Input: part model. Units: mm. Frame: model coordinates. A direction names the side the tool comes from. Round coordinates to 2 decimals unless told otherwise and drop trailing zeros. Write each loop counter-clockwise with the first axis right and the second up, starting at its lowest first coordinate (ties: lowest second). Pieces come first, ordered by that corner, then holes. Notation, with made-up numbers: (5.5, 72) -> (32.5, 72) arc R34 cw to (32.5, 102) -> close; hole circle Ø8 at (-26.75, 72.25). An arc over 180 degrees is marked (long way). Use CSV: the item, a comma, the result in double quotes.
```python
from build123d import *

# Parameters (mm, degrees)
CROQUIS1_W              = 90
CROQUIS1_H              = 53
SALIENTE_EXTRUIR1_DEPTH = 3
CROQUIS2_R              = 1.75
CORTAR_EXTRUIR1_DEPTH   = 53.309177015
CROQUIS3_R              = 3.5
CROQUIS3_R_2            = 1.75
SALIENTE_EXTRUIR2_DEPTH = 3
REDONDEO1_R             = 3
CORTAR_EXTRUIR2_DEPTH   = 53.566624392


with BuildPart() as part:
    # Croquis1 → Saliente-Extruir1 (new body)
    with BuildSketch(Plane(origin=(0, 0, 0), x_dir=(1, 0, 0), z_dir=(0, 1, 0))):
        Rectangle(CROQUIS1_W, CROQUIS1_H)
    extrude(amount=SALIENTE_EXTRUIR1_DEPTH)

    # Croquis2 → Cortar-Extruir1 (cut, through all)
    with BuildSketch(Plane.XZ):
        with Locations(Location((41, -22.5, 0), (0, 0, 270))):
            Circle(CROQUIS2_R)
        with Locations(Location((41, 22.5, 0), (0, 0, 270))):
            Circle(CROQUIS2_R)
        with Locations(Location((-41, 22.5, 0), (0, 0, 270))):
            Circle(CROQUIS2_R)
        with Locations(Location((-41, -22.5, 0), (0, 0, 270))):
            Circle(CROQUIS2_R)
    extrude(amount=-CORTAR_EXTRUIR1_DEPTH, mode=Mode.SUBTRACT)

    # Croquis3 → Saliente-Extruir2 (add)
    # profile 1 of 2: a face of its own
    with BuildSketch(Plane(origin=(0, 3, 0), x_dir=(1, 0, 0), z_dir=(0, 1, 0))):
        with Locations(Location((41, 22.5, 0), (0, 0, 270))):
            Circle(CROQUIS3_R)
        with Locations(Location((41, 22.5, 0), (0, 0, 90))):
            Circle(CROQUIS3_R_2, mode=Mode.SUBTRACT)
    # profile 2 of 2: a face of its own
    with BuildSketch(Plane(origin=(0, 3, 0), x_dir=(1, 0, 0), z_dir=(0, 1, 0))):
        with Locations(Location((-41, 22.5, 0), (0, 0, 270))):
            Circle(CROQUIS3_R)
        with Locations(Location((-41, 22.5, 0), (0, 0, 90))):
            Circle(CROQUIS3_R_2, mode=Mode.SUBTRACT)
    saliente_extruir2 = extrude(amount=SALIENTE_EXTRUIR2_DEPTH)

    # Simetría1: Saliente-Extruir2 across plane
    add(saliente_extruir2.mirror(Plane.XY))

    # Redondeo1
    redondeo1_edges = [part.edges().sort_by_distance(p)[0] for p in [
        (-45, 1.5, -26.5),
        (45, 1.5, -26.5),
        (45, 1.5, 26.5),
        (-45, 1.5, 26.5),
    ]]
    fillet(redondeo1_edges, radius=REDONDEO1_R)

    # Croquis4 → Cortar-Extruir2 (cut, through all)
    with BuildSketch(Plane.XZ):
        Polygon((33.981328373, 21.5), (0, 2.851710039), (-33.981328373, 21.5), align=None)
        Polygon((-40, 19.099509473), (-5.196449405, 0), (-40, -19.099509473), align=None)
        Polygon((40, 19.099509473), (5.196449405, 0), (40, -19.099509473), align=None)
        Polygon((33.981328373, -21.5), (-33.981328373, -21.5), (0, -2.851710039), align=None)
    extrude(amount=-CORTAR_EXTRUIR2_DEPTH, mode=Mode.SUBTRACT)


solid = part.part
```
Item 1: First-contact query: pin 1 Ø5.5 at (x, z) = (-41, -22.5) entering from -Y. Flat tip, straight axial feed; report the tip coordinate or a pass-through.
Worked answers:
pin 1,"stops at y = 0"
Item 2: Section query B-B on x = -41. Return the cut outline in (y, z).
Worked answers:
outline,"(0, -26.5) -> (3, -26.5) -> (3, -26) -> (6, -26) -> (6, -24.25) -> (0, -24.25) -> close; (0, -20.75) -> (6, -20.75) -> (6, -19) -> (3, -19) -> (3, 19) -> (6, 19) -> (6, 20.75) -> (0, 20.75) -> close; (0, 24.25) -> (6, 24.25) -> (6, 26) -> (3, 26) -> (3, 26.5) -> (0, 26.5) -> close"
Item 3: Section query A-A on y = 4.8. Return the cut outline in (x, z).
Worked answers:
outline,"circle Ø7 at (-41, -22.5); circle Ø7 at (-41, 22.5); circle Ø7 at (41, -22.5); circle Ø7 at (41, 22.5); hole circle Ø3.5 at (-41, -22.5); hole circle Ø3.5 at (-41, 22.5); hole circle Ø3.5 at (41, -22.5); hole circle Ø3.5 at (41, 22.5)"
Item 4: Set-up query: faces 4 (the face through (44.1, 1.52, 25.64)), 5 (the face through (-37.53, 4.48, -22.96)), 6 (the face through (-17.229, 1.479, -12.306)). Return all of +Z, -Z, +X, -X, +Y, -Y with unobstructed straight access to the full face (end or side cutting, diameter ignored); none if empty.
Worked answers:
face 4,"+Z, +X, +Y, -Y"
face 5,"+Y"
face 6,"+Y, -Y"
Item 5: Section query C-C on z = 22.5. Return the cut outline in (x, y), plus the area to 3 significant figures.
Worked answers:
outline,"(-45, 0) -> (-42.75, 0) -> (-42.75, 6) -> (-44.5, 6) -> (-44.5, 3) -> (-45, 3) -> close; (-39.25, 0) -> (39.25, 0) -> (39.25, 6) -> (37.5, 6) -> (37.5, 3) -> (-37.5, 3) -> (-37.5, 6) -> (-39.25, 6) -> close; (42.75, 0) -> (45, 0) -> (45, 3) -> (44.5, 3) -> (44.5, 6) -> (42.75, 6) -> close"
area,"270 mm²"
Item 6: Pull-direction query (X, two-part tool) for faces 1 (the face through (-39.254, 2.958, 22.385)), 2 (the face through (-44.14, 1.52, -25.6)), 3 (the face through (43, 6, -22)); classes: +X half, -X half, draft (parallel to the pull), parting line (faces both ways), or undercut.
Worked answers:
face 1,"undercut"
face 2,"-X half"
face 3,"draft"
Item 7: Section query D-D on x = 22.5. Return the cut outline in (y, z), plus the area to 3 significant figures.
Worked answers:
outline,"(0, -26.5) -> (3, -26.5) -> (3, -21.5) -> (0, -21.5) -> close; (0, -15.2) -> (3, -15.2) -> (3, -9.5) -> (0, -9.5) -> close; (0, 9.5) -> (3, 9.5) -> (3, 15.2) -> (0, 15.2) -> close; (0, 21.5) -> (3, 21.5) -> (3, 26.5) -> (0, 26.5) -> close"
area,"64.2 mm²"
Item 8: Line query: line 1 (X direction, y = 1, z = -22.5); line 2 (Z direction, x = 41, y = 1.35); line 3 (X direction, y = 4.2, z = 22.5). Output: solid intervals per line, ascending.
Worked answers:
line 1,"x = -45 to -42.75, -39.25 to 39.25, 42.75 to 45"
line 2,"z = -26.5 to -24.25, -20.75 to 20.75, 24.25 to 26.5"
line 3,"x = -44.5 to -42.75, -39.25 to -37.5, 37.5 to 39.25, 42.75 to 44.5"
